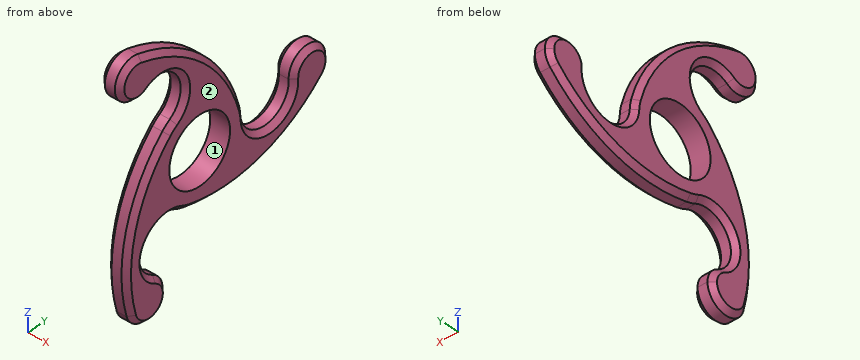
```python
from build123d import *

# Parameters (mm, degrees)
F0_R     = 12.7
F1_DEPTH = 7.62
F2_SIZE  = 1.905


with BuildPart() as f1:
    # F0 (on Right) → F1 (new body)
    with BuildSketch(Plane.YZ):
        with BuildLine():
            ThreePointArc((-4.818668, -18.430489), (11.642742, -15.078099), (19.05, 0))
            ThreePointArc((19.05, 0), (19.042134, 0.547394), (19.018542, 1.094337))
            ThreePointArc((19.018542, 1.094337), (18.798495, 3.085302), (18.370606, 5.042156))
            ThreePointArc((18.370606, 5.042156), (6.727297, 17.822625), (-10.456994, 15.923372))
            ThreePointArc((-10.456994, 15.923372), (-12.071198, 14.737323), (-13.551938, 13.388334))
            ThreePointArc((-13.551938, 13.388334), (-18.798495, -3.085302), (-8.561547, -17.017709))
            ThreePointArc((-8.561547, -17.017709), (-6.727297, -17.822625), (-4.818668, -18.430489))
        make_face()
        Circle(F0_R, mode=Mode.SUBTRACT)
        with BuildLine():
            ThreePointArc((19.018542, 1.094337), (19.042134, 0.547394), (19.05, 0))
            ThreePointArc((19.05, 0), (11.642742, -15.078099), (-4.818668, -18.430489))
            ThreePointArc((-4.818668, -18.430489), (25.888789, -18.218752), (52.350766, -2.638108))
            ThreePointArc((52.350766, -2.638108), (44.233214, -4.434102), (39.304986, 2.26163))
            ThreePointArc((39.304986, 2.26163), (29.74541, -8.465239), (19.018542, 1.094337))
        make_face()
        with BuildLine():
            ThreePointArc((-10.456994, 15.923372), (6.727297, 17.822625), (18.370606, 5.042156))
            ThreePointArc((18.370606, 5.042156), (2.833508, 31.529725), (-23.890715, 46.656147))
            ThreePointArc((-23.890715, 46.656147), (-19.770348, 43.944661), (-18.173919, 39.27765))
            ThreePointArc((-18.173919, 39.27765), (-19.088052, 35.658847), (-21.611122, 32.908302))
            ThreePointArc((-21.611122, 32.908302), (-7.541593, 29.9929), (-10.456994, 15.923372))
        make_face()
        with BuildLine():
            ThreePointArc((54.532403, 2.699364), (46.693445, 10.316218), (39.304986, 2.26163))
            ThreePointArc((39.304986, 2.26163), (44.233214, -4.434102), (52.350766, -2.638108))
            ThreePointArc((52.350766, -2.638108), (53.965938, -0.183696), (54.532403, 2.699364))
        make_face()
        with BuildLine():
            ThreePointArc((-17.693864, -35.169931), (-22.203817, -21.527661), (-8.561547, -17.017709))
            ThreePointArc((-8.561547, -17.017709), (-18.798495, -3.085302), (-13.551938, 13.388334))
            ThreePointArc((-13.551938, 13.388334), (-28.722296, -13.310972), (-28.460051, -44.018039))
            ThreePointArc((-28.460051, -44.018039), (-25.956652, -36.090035), (-17.693864, -35.169931))
        make_face()
        with BuildLine():
            ThreePointArc((-18.173919, 39.27765), (-19.770348, 43.944661), (-23.890715, 46.656147))
            ThreePointArc((-23.890715, 46.656147), (-33.311277, 38.031163), (-21.611122, 32.908302))
            ThreePointArc((-21.611122, 32.908302), (-19.088052, 35.658847), (-18.173919, 39.27765))
        make_face()
        with BuildLine():
            ThreePointArc((-13.498483, -41.977015), (-14.631574, -37.978965), (-17.693864, -35.169931))
            ThreePointArc((-17.693864, -35.169931), (-25.956652, -36.090035), (-28.460051, -44.018039))
            ThreePointArc((-28.460051, -44.018039), (-20.088519, -49.527086), (-13.498483, -41.977015))
        make_face()
    extrude(amount=F1_DEPTH)

    # F2
    f2_edges = [f1.edges().sort_by_distance(p)[0] for p in [
        (0, 25.888789, -18.218752),
        (0, 29.74541, -8.465239),
        (7.62, 25.888789, -18.218752),
    ]]
    chamfer(f2_edges, length=F2_SIZE)


solid = f1.part
```
Check sheet for the modelled part. Datum: model origin and axes. Units: mm. Face numbers are marked on the shaded views. Round coordinates to 2 decimals unless told otherwise and drop trailing zeros. Loops run counter-clockwise (first coordinate to the right, second up) from the corner with the lowest first, then second, coordinate; pieces in that order, holes last. Notation, with made-up numbers: (78.5, -10) - (113.5, -10) arc R20 cw to (113.5, 6) - close; hole circle Ø4 at (10, 57.5). An arc over 180 degrees is marked (long way). Answer as a JSON object with one key per item and string values. Group by question number.
Q1. Scan lines: line 1 along Z through (x, y) = (1, -8); line 2 along Y through (x, z) = (5.5, 8.5); line 3 along Z through (x, y) = (2, 0). Record each from-to range of solid material in increasing order. Write a range as [from, to].
Q2. Mould release check, pull along Z, two halves, no side actions. Record for the marked faces 1 and 2: released by +Z, released by -Z, zero draft, split by the parting line, or undercut.
Q3. Gauge pin test, flat ends, axial feed: P1, Ø4, axis at x = 2, y = 34.5, coming from the +Z side; P2, Ø1, axis at x = 4, y = 4.5, coming from the +Z side; P3, Ø12, axis at y = 23, z = 10, coming from the -X side. Record the tip position at first contact, or that the pin passes through.
Q4. Sectioned sample at A-A, the plane x = 4.5. Enter the section's corners in (y, z), plus the area to 3 significant figures.
Solution:
{
 "1": {"line 1": "z = [-16.29, -9.86], [9.86, 16.81], [32.02, 38.9]", "line 2": "y = [-17.88, -9.44], [9.44, 17.31], [41.97, 51.85]", "line 3": "z = [-19.48, -12.7], [12.7, 34.14]"},
 "2": {"face 1": "undercut", "face 2": "zero draft"},
 "3": {"P1": "stops at z = -5.35", "P2": "stops at z = 30.35", "P3": "stops at x = 1.78"},
 "4": {"outline": "(-28.46, -44.02) arc R7.62 ccw to (-13.5, -41.98) arc R7.62 ccw to (-17.69, -35.17) arc R10.16 cw to (-8.56, -17.02) arc R19.05 ccw to (-4.82, -18.43) arc R59.14 ccw to (52.35, -2.64) arc R7.62 ccw to (54.53, 2.7) arc R7.62 ccw (long way) to (39.3, 2.26) arc R10.16 cw to (19.02, 1.09) arc R19.05 ccw to (18.37, 5.04) arc R59.14 ccw to (-23.89, 46.66) arc R7.62 ccw (long way) to (-21.61, 32.91) arc R10.16 cw to (-10.46, 15.92) arc R19.05 ccw to (-13.55, 13.39) arc R59.14 ccw to start; hole circle Ø25.4 at (0, 0)", "area": "2,290 mm²"}
}
